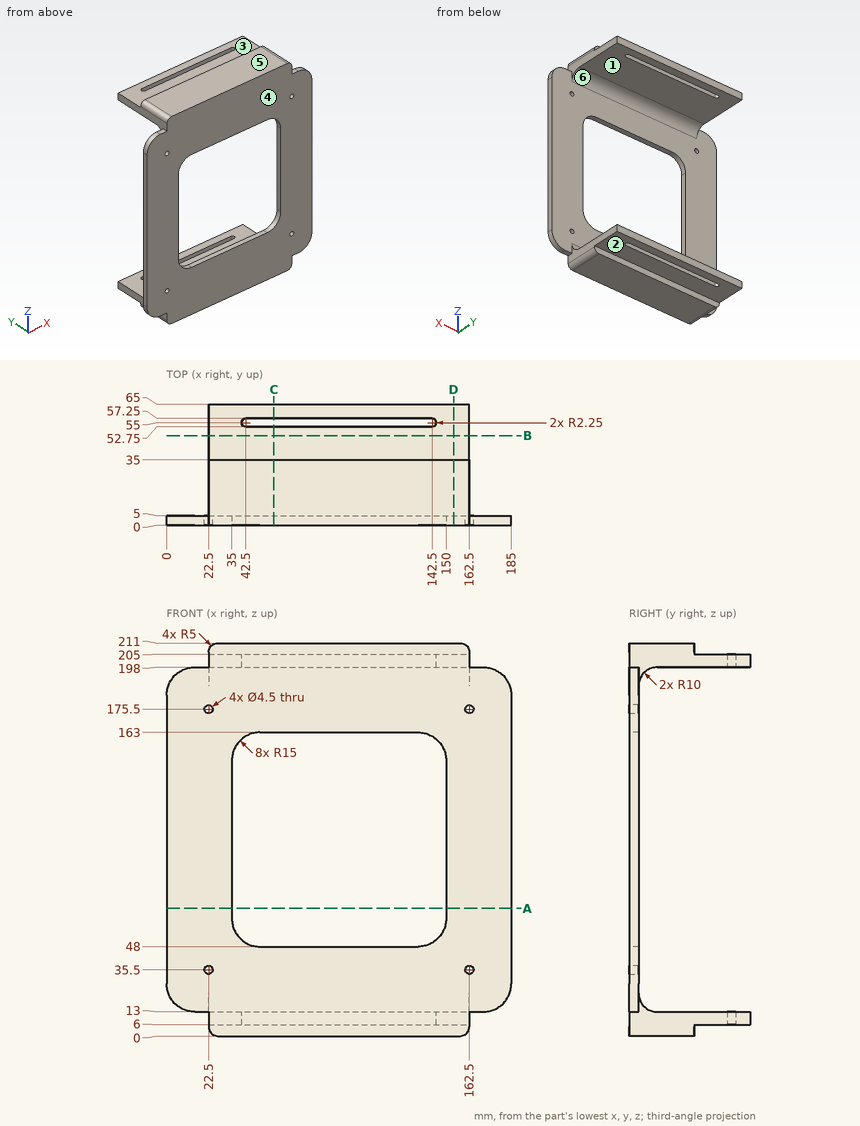
Geometry check sheet. Reference: drawing and pictorial views, mm from the part's lowest x, y, z. A direction names the side the tool comes from. Round coordinates to 2 decimals unless told otherwise and drop trailing zeros. Write each loop counter-clockwise with the first axis right and the second up, starting at its lowest first coordinate (ties: lowest second). Pieces come first, ordered by that corner, then holes.
1. Scan lines: L1, parallel to X at y = 2.1, z = 175.5; L2, parallel to Z at x = 107, y = 20; L3, parallel to Y at x = 120, z = 33.5. Record each from-to range of solid material in increasing order.
2. Access from +Z, -Z, +X, -X, +Y, -Y to the whole of each face (thin tool, end or side, straight path). Record for the marked faces 5 and 6.
3. Section check D-D on x = 154. Enter the section's corners in (y, z), plus the area to 3 significant figures.
4. Section check C-C on x = 57.5. Enter the section's corners in (y, z), plus the area to 3 significant figures.
5. Section check A-A on z = 68.5. Enter the section's corners in (x, y), plus the area to 3 significant figures.
6. Gauge pin test, flat ends, axial feed: P1, Ø20, axis at y = 17, z = 13, coming from the +X side; P2, Ø1.5, axis at x = 17.5, y = 1.5, coming from the -Z side; P3, Ø9, axis at y = 26.5, z = 13.5, coming from the -X side. Record the tip position at first contact, or that the pin passes through.
7. Draft check along Z on the marked faces 1, 2, 3 and 4. Enter one of: +Z half, -Z half, draft (parallel to the pull), parting line (faces both ways), or undercut.
8. Section check B-B on y = 48. Enter the section's corners in (x, z).
Answer:
1. L1: x = 0 to 20.25, 24.75 to 160.25, 164.75 to 185
1. L2: z = 0 to 13, 198 to 211
1. L3: y = 0 to 5
2. face 5: +Z, +X, -X, +Y, -Y
2. face 6: +X, -X, +Y
3. outline: (0, 0) - (35, 0) - (35, 6) - (65, 6) - (65, 13) - (15, 13) arc R10 cw to (5, 23) - (5, 188) arc R10 cw to (15, 198) - (65, 198) - (65, 205) - (35, 205) - (35, 211) - (0, 211) - close
3. area: 2,300 mm2
4. outline: (0, 0) - (35, 0) - (35, 6) - (52.75, 6) - (52.75, 13) - (15, 13) arc R10 cw to (5, 23) - (5, 48) - (0, 48) - close; (0, 163) - (5, 163) - (5, 188) arc R10 cw to (15, 198) - (52.75, 198) - (52.75, 205) - (35, 205) - (35, 211) - (0, 211) - close; (57.25, 6) - (65, 6) - (65, 13) - (57.25, 13) - close; (57.25, 198) - (65, 198) - (65, 205) - (57.25, 205) - close
4. area: 1,660 mm2
5. outline: (0, 0) - (35, 0) - (35, 5) - (0, 5) - close; (150, 0) - (185, 0) - (185, 5) - (150, 5) - close
5. area: 350 mm2
6. P1: stops at x = 162.5
6. P2: stops at z = 13
6. P3: stops at x = 22.5
7. face 1: undercut
7. face 2: -Z half
7. face 3: +Z half
7. face 4: draft
8. outline: (22.5, 6) - (162.5, 6) - (162.5, 13) - (22.5, 13) - close; (22.5, 198) - (162.5, 198) - (162.5, 205) - (22.5, 205) - close
